Check sheet for the modelled part. Datum: model origin and axes. Units: mm. Face numbers are marked on the shaded views. A direction names the side the tool comes from. Give positions to 0.01 mm unless a question says otherwise; leave off trailing zeros. Write each loop counter-clockwise with the first axis right and the second up, starting at its lowest first coordinate (ties: lowest second). Pieces come first, ordered by that corner, then holes. Notation, with made-up numbers: (63, -30) -> (118, -30) arc R21 cw to (118, -19) -> close; hole circle Ø4 at (-1, 4). An arc over 180 degrees is marked (long way). Answer as a JSON object with one key per item and string values.
Autodesk Inventor part; units mm, degrees
ref_plane "YZ Plane" through (0, 0, 0) normal (1, 0, 0) x (0, 1, 0)
ref_plane "XZ Plane" through (0, 0, 0) normal (0, 1, 0) x (-1, 0, 0)
ref_plane "XY Plane" through (0, 0, 0) normal (0, 0, 1) x (1, 0, 0)
sketch "Szkic1" plane through (0, 0, 0) normal (0, 1, 0) x (-1, 0, 0)
  circle A0 centre (0, 0) radius 11.1
  circle A1 centre (0, 0) radius 13.1
  line L0 (-7.5, 20) -> (7.5, 20)
  line L1 (0, 20) -> (0, 0) construction
  line L2 (7.5, 20) -> (12.5093, 3.8895)
  line L3 (-7.5, 20) -> (-12.5093, 3.8895)
  circle A2 centre (0, 16.5) radius 1.75
  line L4 (0, 0) -> (13.1, 0) construction
  line L5 (-7.5, -20) -> (7.5, -20)
  line L6 (0, -20) -> (0, 0) construction
  line L7 (7.5, -20) -> (12.5093, -3.8895)
  line L8 (-7.5, -20) -> (-12.5093, -3.8895)
  circle A3 centre (0, -16.5) radius 1.75
  arc A4 (12.5093, 3.8895) -> (-12.5093, 3.8895) centre (0, 0) ccw
  arc A5 (-12.5093, -3.8895) -> (12.5093, -3.8895) centre (0, 0) ccw
  dimension "d0" = 22.2
  dimension "d1" = 2
  dimension "d2" = 15
  dimension "d3" = 20
  dimension "d7" = 16.5
  dimension "d8" = 3.5
extrude "Wyciągnięcie proste1" add sketch "Szkic1" along normal blind 7
sketch "Szkic2" plane through (0, 7, 0) normal (0, 1, 0) x (1, 0, 0)
  circle A0 centre (0, 0) radius 13.1
  arc A1 (-12.5093, 3.8895) -> (-12.5093, -3.8895) centre (0, 0) ccw construction
  circle A2 centre (0, 0) radius 10.1
  circle A3 centre (0, 0) radius 11.1 construction
  dimension "d16" = 1
extrude "Wyciągnięcie proste2" add sketch "Szkic2" against normal blind 2
fillet "Zaokrąglenie1" radius 5 4 edges at (-7.5, 3.5, 20) (7.5, 3.5, 20) (7.5, 3.5, -20) (-7.5, 3.5, -20)
sketch "Sketch3" plane through (0, 7, 0) normal (0, 1, 0) x (1, 0, 0)
  circle A0 centre (0, 0) radius 10.1
extrude "Extrusion3" add sketch "Sketch3" against normal blind 1
chamfer "Chamfer1" distance 1 angle 45 1 edges at (-10.1, 6, 0)
properties part number "CH_01_0022_bearing_mount"
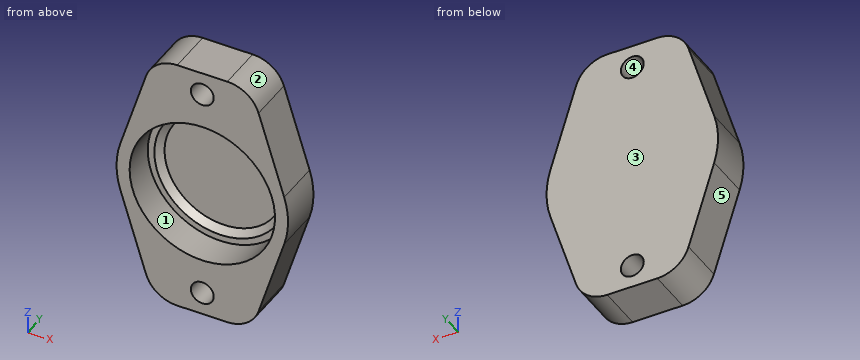
1. Go/stop test with flat-tipped pins: P1, Ø2, axis at y = 1, z = -6, coming from the +X side; P2, Ø6.5, axis at x = 3, z = 2, coming from the -Y side; P3, Ø2, axis at y = 6, z = 6.5, coming from the -X side; P4, Ø2, axis at x = 0, z = 16.5, coming from the -Y side. Record where each tip stops, or that it passes through.
Determined:
{"P1": "x = 12.16", "P2": "y = 6", "P3": "x = -12.01", "P4": "through"}
2. Mould release check, pull along X, two halves, no side actions. Record for the marked faces 3, 4 and 5: released by +X, released by -X, zero draft, split by the parting line, or undercut.
Determined:
{"face 3": "zero draft", "face 4": "undercut", "face 5": "released by -X"}
3. Access from +Z, -Z, +X, -X, +Y, -Y to the whole of each face (thin tool, end or side, straight path). Record for the marked faces 1 and 2.
Determined:
{"face 1": "-Y", "face 2": "+Z, +X, +Y, -Y"}
4. Sectioned sample at B-B, the plane x = 0. State how many separate pieces and enclosed holes the cut face has, plus the area to 3 significant figures.
Determined:
{"separate pieces": "3", "enclosed holes": "0", "area": "101 mm^2"}
5. Sectioned sample at D-D, the plane x = -10.5. Enter the section's corners in (y, z), plus the area to 3 significant figures.
Determined:
{"outline": "(0, -10.35) -> (7, -10.35) -> (7, 10.35) -> (0, 10.35) -> (0, 3.6) -> (5, 3.6) -> (5, -3.6) -> (0, -3.6) -> close", "area": "109 mm^2"}
6. Sectioned sample at A-A, the plane y = 1.5. Enter the section's corners in (x, z).
Determined:
{"outline": "(-12.51, -3.89) -> (-8.59, -16.48) arc R5 ccw to (-3.82, -20) -> (3.82, -20) arc R5 ccw to (8.59, -16.48) -> (12.51, -3.89) arc R13.1 ccw to (12.51, 3.89) -> (8.59, 16.48) arc R5 ccw to (3.82, 20) -> (-3.82, 20) arc R5 ccw to (-8.59, 16.48) -> (-12.51, 3.89) arc R13.1 ccw to start; hole circle Ø22.2 at (0, 0); hole circle Ø3.5 at (0, -16.5); hole circle Ø3.5 at (0, 16.5)"}
7. Scan lines: L1, parallel to Z at x = 0, y = 4; L2, parallel to X at y = 1.15, z = 0; L3, parallel to Z at x = 0, y = 5.75. Record each from-to range of solid material in increasing order. Write a range as [from, to].
Determined:
{"L1": "[-20, -18.25], [-14.75, -11.1], [11.1, 14.75], [18.25, 20]", "L2": "[-13.1, -11.1], [11.1, 13.1]", "L3": "[-20, -18.25], [-14.75, -9.35], [9.35, 14.75], [18.25, 20]"}
